Read the model definition and answer for the solid it produces. Units are mm, in the model's axes. A direction names the side the tool comes from. Round coordinates to 2 decimals unless told otherwise and drop trailing zeros. Loops run counter-clockwise (first coordinate to the right, second up) from the corner with the lowest first, then second, coordinate; pieces in that order, holes last. Notation, with made-up numbers: (-9, 73.5) -> (10, 73.5) arc R18 cw to (10, 99.5) -> close; hole circle Ø7 at (-39.75, -4). An arc over 180 degrees is marked (long way). Put each result on its own line as item: value.
from build123d import *

# Parameters (mm, degrees)
BASPROSKE_W        = 10
BASPROSKE_H        = 16
TOOTHCUT_DEPTH     = 25.738633754
TEETHCUTS_COUNT    = 30
TEETHCUTS_ANGLE    = 348
HUBNEAONESKE_R     = 12.5
HUBNEARONE_DEPTH   = 8.0000508
BORSKE_R           = 3
BORE_DEPTH         = 18.0000508
SKETCH2_R          = 12.5
CUT_EXTRUDE1_DEPTH = 8.0000508
SKETCH3_R          = 5.1
CUT_EXTRUDE2_DEPTH = 10
SKETCH4_R          = 1.5
CUT_EXTRUDE3_DEPTH = 10


with BuildPart() as part:
    # BasProSke → Base-Revolve (revolve)
    with BuildSketch(Plane(origin=(0, 0, 0), x_dir=(1, 0, 0), z_dir=(0, 1, 0)), mode=Mode.PRIVATE) as base_revolve_sk:
        with Locations((5, 8)):
            Rectangle(BASPROSKE_W, BASPROSKE_H)
    revolve(base_revolve_sk.sketch.rotate(Axis((-10, 0, 0), (1, 0, 0)), 180), axis=Axis((-10, 0, 0), (1, 0, 0)))

    # TooCutSke → ToothCut (cut, through all)
    with BuildSketch(Plane(origin=(0, 0, 0), x_dir=(0, 0, -1), z_dir=(1, 0, 0))):
        with BuildLine():
            ThreePointArc((0.466400716, 13.741086979), (0, 13.749), (-0.466400716, 13.741086979))
            ThreePointArc((-0.466400716, 13.741086979), (-0.819142092, 14.899954875), (-1.3974676, 15.964351834))
            ThreePointArc((-1.3974676, 15.964351834), (0, 16.0254), (1.3974676, 15.964351834))
            ThreePointArc((1.3974676, 15.964351834), (0.819142092, 14.899954875), (0.466400716, 13.741086979))
        make_face()
    toothcut = extrude(amount=TOOTHCUT_DEPTH, mode=Mode.SUBTRACT)

    # TeethCuts: ToothCut ×30 about axis
    teethcuts_axis = Axis((-10, 0, 0), (1, 0, 0))
    for i in range(1, TEETHCUTS_COUNT):
        add(toothcut.rotate(teethcuts_axis, i * TEETHCUTS_ANGLE / (TEETHCUTS_COUNT - 1)), mode=Mode.SUBTRACT)

    # HubNeaOneSke → HubNearOne (add)
    with BuildSketch(Plane.ZY):
        with Locations(Location((0, 0, 0), (0, 0, 180))):
            Circle(HUBNEAONESKE_R)
    extrude(amount=HUBNEARONE_DEPTH)

    # BorSke → Bore (cut, symmetric)
    with BuildSketch(Plane(origin=(0, 0, 0), x_dir=(0, 0, -1), z_dir=(1, 0, 0))):
        with Locations(Location((0, 0, 0), (0, 0, 180))):
            Circle(BORSKE_R)
    extrude(amount=BORE_DEPTH, both=True, mode=Mode.SUBTRACT)

    # Sketch2 → Cut-Extrude1 (cut)
    with BuildSketch(Plane.ZY.offset(8.0000508)):
        Circle(SKETCH2_R)
    extrude(amount=-CUT_EXTRUDE1_DEPTH, mode=Mode.SUBTRACT)

    # Sketch3 → Cut-Extrude2 (cut)
    with BuildSketch(Plane(origin=(10, 0, 0), x_dir=(0, 0, -1), z_dir=(1, 0, 0))):
        Circle(SKETCH3_R)
    extrude(amount=-CUT_EXTRUDE2_DEPTH, mode=Mode.SUBTRACT)

    # Sketch4 → Cut-Extrude3 (cut)
    with BuildSketch(Plane.ZY):
        with BuildLine():
            ThreePointArc((-4.243347723, 2.829134161), (-3.606244584, 3.606244584), (-2.829134161, 4.243347723))
            Line((-2.829134161, 4.243347723), (-3.535533906, 4.949747468))
            Line((-3.535533906, 4.949747468), (-4.949747468, 3.535533906))
            Line((-4.949747468, 3.535533906), (-4.243347723, 2.829134161))
        make_face()
        with Locations((0, -8)):
            Circle(SKETCH4_R)
        with Locations((8, 0)):
            Circle(SKETCH4_R)
        with Locations((-8, 0)):
            Circle(SKETCH4_R)
        with Locations((0, 8)):
            Circle(SKETCH4_R)
    extrude(amount=-CUT_EXTRUDE3_DEPTH, mode=Mode.SUBTRACT)


solid = part.part
Item 1: The part is cut by section B-B (x = 8.5). State how many separate pieces and enclosed holes the cut face has, then the cut area to 3 significant figures.
Derived:
separate pieces: 1
enclosed holes: 5
area: 579 mm^2
Item 2: Which of the six approach directions +Z, -Z, +X, -X, +Y, -Y give full straight-line access (tool end or side, diameter ignored) to faces 1 (the cylindrical face through (4.93, -11.574, 9.423)), 2 (the cylindrical face through (4.93, -9.36, 11.62)), 3 (the cylindrical face through (4.93, 0.74, -14.91))?
Derived:
face 1: +X, -X, -Y
face 2: +X, -X
face 3: -Z, +X, -X
Item 3: The part is cut by section A-A (y = -8). Determine the outline of the cut face in (x, z), then the cut area to 3 significant figures.
Derived:
outline: (0, -12.37) -> (10, -12.37) -> (10, -1.5) -> (0, -1.5) -> close; (0, 1.5) -> (10, 1.5) -> (10, 12.37) -> (0, 12.37) -> close
area: 217 mm^2
Item 4: Find the intervals of material crossed by line 1 along Y through (x, z) = (6.5, -10); line 2 along Y through (x, z) = (5.5, -12.5); line 3 along Z through (x, y) = (4.75, 15), in increasing order.
Derived:
line 1: y = -11.88 to -9.68, -9.44 to 9.44, 9.68 to 11.88
line 2: y = -9.6 to -8.17, -6.58 to 6.58, 8.17 to 9.6
line 3: z = -5.24 to -4.37, -2.24 to -0.86, 0.86 to 2.24, 4.37 to 5.24
Item 5: For a pull along Y with two mould halves and no side action, classify faces 4 (the cylindrical face through (4.93, 0.07, 6.5)), 5 (the cylindrical face through (4.93, -14.406, 3.9)), 6 (the cylindrical face through (4.93, 14.378, 3.881)) as pulls with the +Y half, pulls with the -Y half, needs draft (parallel to the pull), parting line crosses it, or undercut.
Derived:
face 4: undercut
face 5: pulls with the -Y half
face 6: pulls with the +Y half
Item 6: Flat-ended cylindrical pins translate along their axes: pin 1 Ø2.5 at (y, z) = (0, 8) entering from +X; pin 2 Ø11.5 at (y, z) = (0, 0) entering from +X; pin 3 Ø6 at (x, y) = (6.5, 11.5) entering from -Z; pin 4 Ø1.5 at (x, z) = (2, 6.5) entering from +Y. Find the tip coordinate at first contact, or state that the pin passes through.
Derived:
pin 1: passes through
pin 2: stops at x = 10
pin 3: stops at z = -13.11
pin 4: stops at y = 13.66
